The listing builds one solid part. Answer for the finished solid, in the listing's coordinates (mm). A direction names the side the tool comes from. Round coordinates to 2 decimals unless told otherwise and drop trailing zeros. Loops run counter-clockwise (first coordinate to the right, second up) from the corner with the lowest first, then second, coordinate; pieces in that order, holes last. Notation, with made-up numbers: M 14,3 L 29,3 A23 ccw 29,31 Z; hole C 60,65 d6. An arc over 180 degrees is marked long. Put each result on its own line as item: value. Start each with the question number.
(1) Which of the six approach directions +Z, -Z, +X, -X, +Y, -Y give full straight-line access (tool end or side, diameter ignored) to faces 1 (the face through (-2, 512, -36.5)), 2 (the face through (-136.654, 290.128, -155.453)), 3 (the face through (177, 38, -98.5))?
(2) Section C-C, the plane x = -111.5 is taken. Determine the outline of the cut face in (y, z), then the cut area to 3 significant figures.
(3) Determine the mould class of faces 4 (the face through (-125.5, 305, -154)), 5 (the face through (197.5, 301, -123)), 6 (the face through (-177, 117.5, 1)), 7 (the face through (147.5, 312, -167)) for opening direction X: released by +X, released by -X, zero draft, split by the parting line, or undercut.
(4) Flat-ended cylindrical pins translate along their axes: P1, Ø12, axis at x = -168, y = 158.5, coming from the -Z side; P2, Ø6, axis at x = -85.5, y = 492.5, coming from the -Z side; P3, Ø11, axis at x = 150, y = 292.5, coming from the +Z side. Find the tip coordinate at first contact, or state that the pin passes through.
(5) Section B-B, the plane y = 360 is taken. Determine the outline of the cut face in (x, z).
(6) Straight lines are drawn through the part: line 1 (X direction, y = 526, z = 106.5); line 2 (Y direction, x = -172, z = -73.5); line 3 (Y direction, x = -55.5, z = -21). For each, find the intervals that lie inside material, in ascending order.
(7) Section A-A, the plane z = -120 is taken. Determine the outline of the cut face in (x, y).
```python
from build123d import *

# Parameters (mm, degrees)
SKETCH1_W                = 40
SKETCH1_H                = 40
BOSS_EXTRUDE1_DEPTH      = 610
BOSS_EXTRUDE1_2_DEPTH    = 610
BOSS_EXTRUDE1_3_DEPTH    = 610
BOSS_EXTRUDE1_4_DEPTH    = 610
SKETCH2_W                = 40
SKETCH2_H                = 40
BOSS_EXTRUDE2_DEPTH      = 237
BOSS_EXTRUDE3_REACH      = 721.241
SKETCH3_W                = 40
SKETCH3_H                = 40
SKETCH4_W                = 50
SKETCH4_H                = 72
BOSS_EXTRUDE4_DEPTH      = 40
CHAMFER1_SIZE            = 30
SKETCH5_R                = 15
BOSS_EXTRUDE5_DEPTH      = 22
CHAMFER1_OF_MIRROR1_SIZE = 30


with BuildPart() as part:
    # Sketch1 → Boss-Extrude1 (new body)
    with BuildSketch(Plane(origin=(0, 0, 0), x_dir=(1, 0, 0), z_dir=(0, 1, 0))):
        with Locations((-177.5, 118.5)):
            Rectangle(SKETCH1_W, SKETCH1_H)
    extrude(amount=BOSS_EXTRUDE1_DEPTH)



with BuildPart() as body_2:
    # Sketch1 → Boss-Extrude1 2 (new body)
    with BuildSketch(Plane(origin=(0, 0, 0), x_dir=(1, 0, 0), z_dir=(0, 1, 0))):
        with Locations((177.5, 118.5)):
            Rectangle(SKETCH1_W, SKETCH1_H)
    extrude(amount=BOSS_EXTRUDE1_2_DEPTH)


with BuildPart() as body_3:
    # Sketch1 → Boss-Extrude1 3 (new body)
    with BuildSketch(Plane(origin=(0, 0, 0), x_dir=(1, 0, 0), z_dir=(0, 1, 0))):
        with Locations((177.5, -118.5)):
            Rectangle(SKETCH1_W, SKETCH1_H)
    extrude(amount=BOSS_EXTRUDE1_3_DEPTH)


with BuildPart() as body_4:
    # Sketch1 → Boss-Extrude1 4 (new body)
    with BuildSketch(Plane(origin=(0, 0, 0), x_dir=(1, 0, 0), z_dir=(0, 1, 0))):
        with Locations((-177.5, -118.5)):
            Rectangle(SKETCH1_W, SKETCH1_H)
    extrude(amount=BOSS_EXTRUDE1_4_DEPTH)


with BuildPart() as part_1:
    add(part.part)

    add(body_2.part)  # Boss-Extrude2 merges body 2

    add(body_3.part)  # Boss-Extrude2 merges body 3

    add(body_4.part)  # Boss-Extrude2 merges body 4
    # Sketch2 → Boss-Extrude2 (add)
    with BuildSketch(Plane(origin=(0, 0, 98.5), x_dir=(-1, 0, 0), z_dir=(0, 0, -1))):
        with Locations((177.5, 97.5)):
            Rectangle(SKETCH2_W, SKETCH2_H)
        with Locations((-177.5, 97.5)):
            Rectangle(SKETCH2_W, SKETCH2_H)
        with Locations((-177.5, 512.5)):
            Rectangle(SKETCH2_W, SKETCH2_H)
        with Locations((177.5, 512.5)):
            Rectangle(SKETCH2_W, SKETCH2_H)
    extrude(amount=BOSS_EXTRUDE2_DEPTH)

    # Sketch3 → Boss-Extrude3 (add, up to next)
    with BuildSketch(Plane(origin=(-157.5, 0, 0), x_dir=(0, 0, -1), z_dir=(1, 0, 0)), mode=Mode.PRIVATE) as boss_extrude3_sk1:
        with Locations((16.5, 512.5)):
            Rectangle(SKETCH3_W, SKETCH3_H)
    boss_extrude3_tool1 = extrude(boss_extrude3_sk1.sketch, amount=BOSS_EXTRUDE3_REACH, mode=Mode.PRIVATE) - part_1.part
    add(boss_extrude3_tool1.solids().sort_by_distance((-157.5, 512.5, -16.5))[0])

    # Sketch4 → Boss-Extrude4 (add)
    with BuildSketch(Plane(origin=(0, 0, -138.5), x_dir=(-1, 0, 0), z_dir=(0, 0, -1))):
        with Locations((172.5, 305)):
            Rectangle(SKETCH4_W, SKETCH4_H)
    boss_extrude4 = extrude(amount=BOSS_EXTRUDE4_DEPTH)

    # Chamfer1
    chamfer1_edges = [part_1.edges().sort_by_distance(p)[0] for p in [
        (-172.5, 341, -178.5),
        (-172.5, 269, -178.5),
    ]]
    chamfer(chamfer1_edges, length=CHAMFER1_SIZE)

    # Sketch5 → Boss-Extrude5 (add)
    with BuildSketch(Plane(origin=(-147.5, 0, 0), x_dir=(0, 0, -1), z_dir=(1, 0, 0))):
        with Locations(Location((153.5, 305, 0), (0, 0, 180))):
            Circle(SKETCH5_R)
    boss_extrude5 = extrude(amount=BOSS_EXTRUDE5_DEPTH)

    # Mirror1: Boss-Extrude4, Boss-Extrude5 across plane
    add(boss_extrude4.mirror(Plane(origin=(0, 0, 0), x_dir=(0, 0, 1), z_dir=(1, 0, 0))))
    add(boss_extrude5.mirror(Plane(origin=(0, 0, 0), x_dir=(0, 0, 1), z_dir=(1, 0, 0))))

    # Chamfer1 of Mirror1
    chamfer1_of_mirror1_edges = [part_1.edges().sort_by_distance(p)[0] for p in [
        (172.5, 341, -178.5),
        (172.5, 269, -178.5),
    ]]
    chamfer(chamfer1_of_mirror1_edges, length=CHAMFER1_OF_MIRROR1_SIZE)


solid = part_1.part
```
Recorded:
1. face 1: -Z, +Y, -Y
1. face 2: none
1. face 3: +X, -X, -Y
2. outline: M 492.5,-36.5 L 532.5,-36.5 L 532.5,3.5 L 492.5,3.5 Z
2. area: 1,600 mm²
3. face 4: undercut
3. face 5: released by +X
3. face 6: zero draft
3. face 7: undercut
4. P1: stops at z = -138.5
4. P2: stops at z = -36.5
4. P3: stops at z = -138.5
5. outline: M -197.5,-138.5 L -157.5,-138.5 L -157.5,-98.5 L -197.5,-98.5 Z; M -197.5,98.5 L -157.5,98.5 L -157.5,138.5 L -197.5,138.5 Z; M 157.5,-138.5 L 197.5,-138.5 L 197.5,-98.5 L 157.5,-98.5 Z; M 157.5,98.5 L 197.5,98.5 L 197.5,138.5 L 157.5,138.5 Z
6. line 1: x = -197.5 to -157.5, 157.5 to 197.5
6. line 2: y = 77.5 to 117.5, 492.5 to 532.5
6. line 3: y = 492.5 to 532.5
7. outline: M -197.5,0 L -157.5,0 L -157.5,610 L -197.5,610 Z; M 157.5,0 L 197.5,0 L 197.5,610 L 157.5,610 Z
